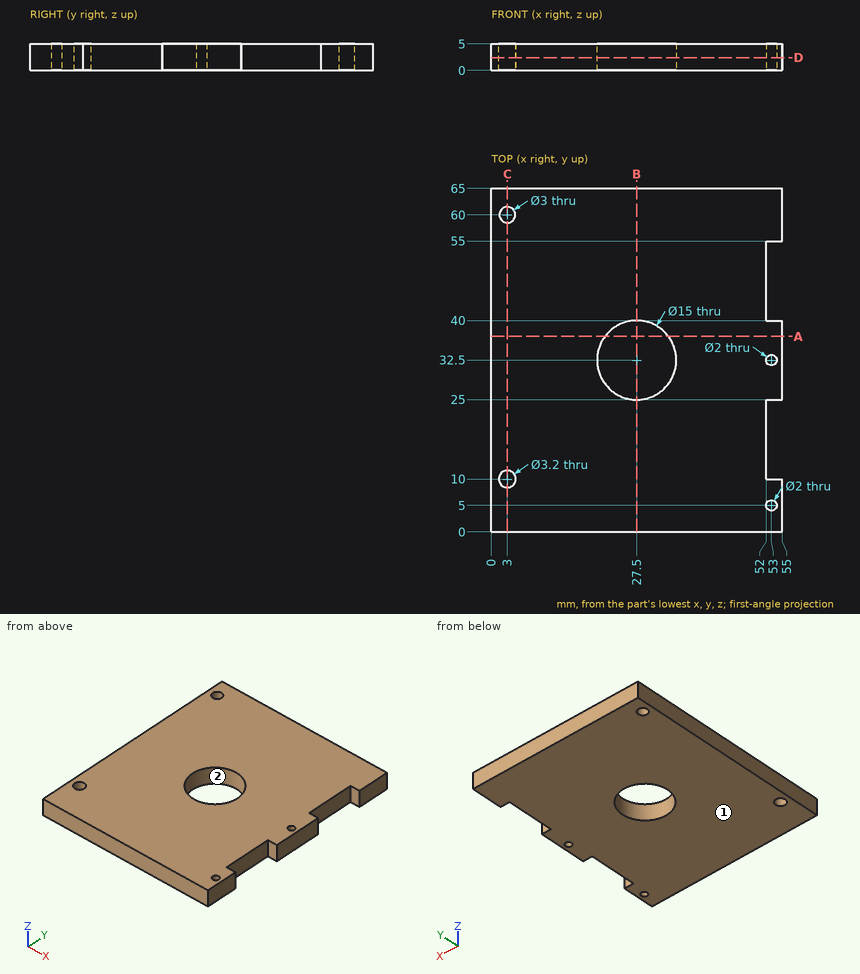
Job drawing, mm, ordinate dimensions from the low corner. One solid piece. Give positions to 0.01 mm unless a question says otherwise; leave off trailing zeros. Loops run counter-clockwise (first coordinate to the right, second up) from the corner with the lowest first, then second, coordinate; pieces in that order, holes last. Notation, with made-up numbers: M 35.5,-21 L 91.5,-21 A24 cw 91.5,-3 Z; hole C 76,-21.5 d3. An arc over 180 degrees is marked long. Return JSON: item names as keys, results as strings.
1) Flat gauge pin, fed straight in: pin 1 Ø1.5 at (x, z) = (53, 3.5) entering from -Y. Where does the tip first touch, or does it go through?
Calculated:
{"pin 1": "stops at y = 0"}
2) Drill centre lines: line 1 (X direction, y = 33, z = 4.35); line 2 (Y direction, x = 3, z = 1.15); line 3 (Y direction, x = 21, z = 4.1). Where is each one in solid material? Low to high.
Calculated:
{"line 1": "x = 0 to 20.02, 34.98 to 52.13, 53.87 to 55", "line 2": "y = 0 to 8.4, 11.6 to 58.5, 61.5 to 65", "line 3": "y = 0 to 28.76, 36.24 to 65"}
3) Saw through at B-B, the plane x = 27.5. List the corners of the cut face in (y, z).
Calculated:
{"outline": "M 0,0 L 25,0 L 25,5 L 0,5 Z; M 40,0 L 65,0 L 65,5 L 40,5 Z"}
4) Saw through at A-A, the plane y = 37. List the corners of the cut face in (x, z).
Calculated:
{"outline": "M 0,0 L 21.5,0 L 21.5,5 L 0,5 Z; M 33.5,0 L 55,0 L 55,5 L 33.5,5 Z"}
5) Pull direction X, two halves, no side cores. Call the marked faces 1 and 2: released by +X, released by -X, zero draft, split by the parting line, or undercut.
Calculated:
{"face 1": "zero draft", "face 2": "undercut"}
6) Saw through at D-D, the plane z = 2.4. List the corners of the cut face in (x, y).
Calculated:
{"outline": "M 0,0 L 55,0 L 55,10 L 52,10 L 52,25 L 55,25 L 55,40 L 52,40 L 52,55 L 55,55 L 55,65 L 0,65 Z; hole C 3,10 d3.2; hole C 3,60 d3; hole C 27.5,32.5 d15; hole C 53,5 d2; hole C 53,32.5 d2"}
7) Saw through at C-C, the plane x = 3. List the corners of the cut face in (y, z), then the cut area to 3 significant figures.
Calculated:
{"outline": "M 0,0 L 8.4,0 L 8.4,5 L 0,5 Z; M 11.6,0 L 58.5,0 L 58.5,5 L 11.6,5 Z; M 61.5,0 L 65,0 L 65,5 L 61.5,5 Z", "area": "294 mm2"}
